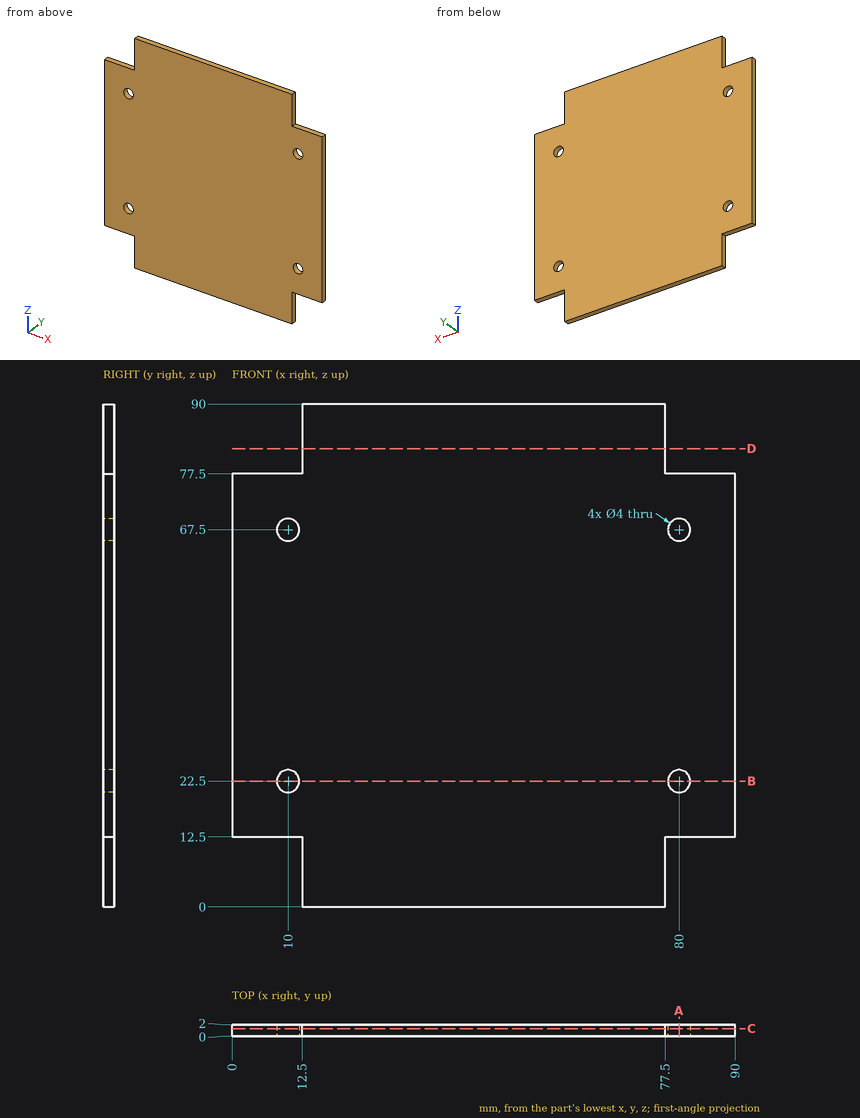
Study the drawing (mm; zero at the part's minimum x, y, z) and answer. Round coordinates to 2 decimals unless told otherwise and drop trailing zeros. Order: outer loops, then holes, each group sorted by start corner. A loop starts at its lowest first (then second) coordinate and runs counter-clockwise, first axis right, second up. Notation, with made-up numbers: M 56,-33 L 90,-33 A17 cw 90,-1 Z; hole C 62,65.5 d7. An arc over 180 degrees is marked long. One line per item, written item: value.
Q1. Find section D-D on z = 82. Write down the section's boundary in (x, y), then the cut area to 3 significant figures.
Derived:
outline: M 12.5,0 L 77.5,0 L 77.5,2 L 12.5,2 Z
area: 130 mm²
Q2. Find section C-C on y = 1.3. Write down the section's boundary in (x, z), then the cut area to 3 significant figures.
Derived:
outline: M 0,12.5 L 12.5,12.5 L 12.5,0 L 77.5,0 L 77.5,12.5 L 90,12.5 L 90,77.5 L 77.5,77.5 L 77.5,90 L 12.5,90 L 12.5,77.5 L 0,77.5 Z; hole C 10,22.5 d4; hole C 10,67.5 d4; hole C 80,22.5 d4; hole C 80,67.5 d4
area: 7,420 mm²
Q3. Find section A-A on x = 80. Write down the section's boundary in (y, z), then the cut area to 3 significant figures.
Derived:
outline: M 0,12.5 L 2,12.5 L 2,20.5 L 0,20.5 Z; M 0,24.5 L 2,24.5 L 2,65.5 L 0,65.5 Z; M 0,69.5 L 2,69.5 L 2,77.5 L 0,77.5 Z
area: 114 mm²
Q4. Find section B-B on z = 22.5. Write down the section's boundary in (x, y), then the cut area to 3 significant figures.
Derived:
outline: M 0,0 L 8,0 L 8,2 L 0,2 Z; M 12,0 L 78,0 L 78,2 L 12,2 Z; M 82,0 L 90,0 L 90,2 L 82,2 Z
area: 164 mm²
Q5. Flat-ended cylindrical pins translate along their axes: pin 1 (0.6 mm diameter, centred on y = 1, z = 6, fed in from -X); pin 2 (0.6 mm diameter, centred on x = 82, y = 1, fed in from +Z); pin 3 (2.5 mm diameter, centred on x = 10, z = 67.5, fed in from +Y); pin 4 (0.6 mm diameter, centred on x = 3.5, y = 1, fed in from -Z). Find the tip coordinate at first contact, or state that the pin passes through.
Derived:
pin 1: x = 12.5
pin 2: z = 77.5
pin 3: through
pin 4: z = 12.5
Q6. Straight lines are drawn through the part: line 1 (X direction, y = 0.8, z = 22.5); line 2 (Z direction, x = 10, y = 0.6); line 3 (X direction, y = 0.2, z = 69). For each, find the intervals that lie inside material, in ascending order.
Derived:
line 1: 0 to 8, 12 to 78, 82 to 90
line 2: 12.5 to 20.5, 24.5 to 65.5, 69.5 to 77.5
line 3: 0 to 8.68, 11.32 to 78.68, 81.32 to 90
